```python
from build123d import *

# Parameters (mm, degrees)
SKETCH1_W           = 12.5
SKETCH1_H           = 10
BOSS_EXTRUDE1_DEPTH = 10
SKETCH2_W           = 10
SKETCH2_H           = 10
BOSS_EXTRUDE2_DEPTH = 5
SKETCH3_R           = 3.5
BOSS_EXTRUDE3_DEPTH = 30
SKETCH4_W           = 4
SKETCH4_H           = 10
CUT_EXTRUDE1_DEPTH  = 11
SKETCH5_W           = 9.5
SKETCH5_H           = 10
BOSS_EXTRUDE4_DEPTH = 12.5
SKETCH6_W           = 5
SKETCH6_H           = 10
BOSS_EXTRUDE5_DEPTH = 30
SKETCH7_R           = 1.75
CUT_EXTRUDE2_DEPTH  = 23.5


with BuildPart() as part:
    # Sketch1 → Boss-Extrude1 (new body)
    with BuildSketch(Plane.XY):
        with Locations((6.25, 5)):
            Rectangle(SKETCH1_W, SKETCH1_H)
    extrude(amount=BOSS_EXTRUDE1_DEPTH)

    # Sketch2 → Boss-Extrude2 (add)
    with BuildSketch(Plane.ZY):
        with Locations((5, 5)):
            Rectangle(SKETCH2_W, SKETCH2_H)
    extrude(amount=BOSS_EXTRUDE2_DEPTH)

    # Sketch3 → Boss-Extrude3 (add)
    with BuildSketch(Plane(origin=(0, 10, 0), x_dir=(1, 0, 0), z_dir=(0, 1, 0))):
        with Locations((3.75, -5)):
            Circle(SKETCH3_R)
    extrude(amount=BOSS_EXTRUDE3_DEPTH)

    # Sketch4 → Cut-Extrude1 (cut, through all)
    with BuildSketch(Plane(origin=(0, 10, 0), x_dir=(1, 0, 0), z_dir=(0, 1, 0))):
        with Locations((10.5, -5)):
            Rectangle(SKETCH4_W, SKETCH4_H)
        with Locations((-3, -5)):
            Rectangle(SKETCH4_W, SKETCH4_H)
    extrude(amount=-CUT_EXTRUDE1_DEPTH, mode=Mode.SUBTRACT)

    # Sketch5 → Boss-Extrude4 (add)
    with BuildSketch(Plane.XY.offset(10)):
        with Locations((3.75, 5)):
            Rectangle(SKETCH5_W, SKETCH5_H)
    extrude(amount=BOSS_EXTRUDE4_DEPTH)

    # Sketch6 → Boss-Extrude5 (add)
    with BuildSketch(Plane(origin=(8.5, 0, 0), x_dir=(0, 0, -1), z_dir=(1, 0, 0))):
        with Locations((-20, 5)):
            Rectangle(SKETCH6_W, SKETCH6_H)
    extrude(amount=BOSS_EXTRUDE5_DEPTH)

    # Sketch7 → Cut-Extrude2 (cut, through all)
    with BuildSketch(Plane.XY.offset(22.5)):
        with Locations((22.5, 5)):
            Circle(SKETCH7_R)
        with Locations((33.5, 5)):
            Circle(SKETCH7_R)
    extrude(amount=-CUT_EXTRUDE2_DEPTH, mode=Mode.SUBTRACT)


solid = part.part
```
The model under review builds one solid part; all positions refer to its coordinate system, in mm. A direction names the side the tool comes from. Round coordinates to 2 decimals unless told otherwise and drop trailing zeros. Write each loop counter-clockwise with the first axis right and the second up, starting at its lowest first coordinate (ties: lowest second). Pieces come first, ordered by that corner, then holes. Notation, with made-up numbers: (9, 77) - (50, 77) arc R13 cw to (50, 82) - close; hole circle Ø7 at (-36.75, -9.5). An arc over 180 degrees is marked (long way). One line per question, with ' | ' between items.
Item 1: To check wall thickness, follow probe 1 along Y at (x, z) = (22.5, 19.8); probe 2 along Z at (x, y) = (20.5, 9.5); probe 3 along Y at (x, z) = (28, 19). State the ranges of each line that lie inside material, in increasing order.
Resolved:
probe 1: y = 0 to 3.25, 6.75 to 10 | probe 2: z = 17.5 to 22.5 | probe 3: y = 0 to 10
Item 2: Add section D-D, the plane z = 19.5. Give the boundary of the cut face in (x, y), then the cut area to 3 significant figures.
Resolved:
outline: (-1, 0) - (38.5, 0) - (38.5, 10) - (-1, 10) - close; hole circle Ø3.5 at (22.5, 5); hole circle Ø3.5 at (33.5, 5) | area: 376 mm2
Item 3: Add section B-B, the plane x = 22.5. Give the boundary of the cut face in (y, z).
Resolved:
outline: (0, 17.5) - (3.25, 17.5) - (3.25, 22.5) - (0, 22.5) - close; (6.75, 17.5) - (10, 17.5) - (10, 22.5) - (6.75, 22.5) - close
Item 4: Add section A-A, the plane y = 5. Give the boundary of the cut face in (x, z).
Resolved:
outline: (-1, 0) - (8.5, 0) - (8.5, 17.5) - (20.75, 17.5) - (20.75, 22.5) - (-1, 22.5) - close; (24.25, 17.5) - (31.75, 17.5) - (31.75, 22.5) - (24.25, 22.5) - close; (35.25, 17.5) - (38.5, 17.5) - (38.5, 22.5) - (35.25, 22.5) - close
Item 5: Add section C-C, the plane z = 5. Give the boundary of the cut face in (x, y), then the cut area to 3 significant figures.
Resolved:
outline: (-1, 0) - (8.5, 0) - (8.5, 10) - (7.25, 10) - (7.25, 40) - (0.25, 40) - (0.25, 10) - (-1, 10) - close | area: 305 mm2
Item 6: For P1, Ø4.5, axis at x = 33.5, y = 5, coming from the -Z side; P2, Ø1, axis at y = 22.5, z = 3, coming from the +X side; P3, Ø4, axis at x = 7, z = 11, coming from the +Y side; P4, Ø3, axis at x = 22.5, y = 5, coming from the +Z side, all flat-tipped, find the tip position at first contact; note any pin that passes through.
Resolved:
P1: stops at z = 17.5 | P2: stops at x = 6.91 | P3: stops at y = 10 | P4: passes through
Item 7: For faces 5 (the face through (7, 24.8, 6.3)), 6 (the face through (10, 0, 19)), 7 (the face through (23, 7, 17.5)), list the 3-axis set-ups (+Z, -Z, +X, -X, +Y, -Y) from which the entire face can be reached by the end or side of a thin tool; tool diameter is ignored.
Resolved:
face 5: +Y | face 6: +Z, -Z, +X, -X, -Y | face 7: -Z, +X, +Y, -Y
Item 8: The part is to be moulded in two halves that separate along Y. For faces 1 (the face through (8.5, 5, 9)), 2 (the face through (31.75, 5.08, 20.04)), 3 (the face through (4, 40, 5)), 4 (the face through (20.75, 5.08, 20.04)), say which applies: pulls with the +Y half, pulls with the -Y half, needs draft (parallel to the pull), parting line crosses it, or undercut.
Resolved:
face 1: needs draft | face 2: undercut | face 3: pulls with the +Y half | face 4: undercut
